from build123d import *

# Parameters (mm, degrees)
SKETCH_1_W          = 66
SKETCH_1_H          = 80
EXTRUDE_1_DEPTH     = 6
SKETCH_2_W          = 41.2
SKETCH_2_H          = 64.2
CUT_EXTRUDE_1_DEPTH = 3
FILLET_1_R          = 1
SKETCH_3_R          = 2.1
CUT_EXTRUDE_2_DEPTH = 53.201532545
CHAMFER_1_SIZE      = 1
FILLET_2_R          = 20
FILLET_3_R          = 10
CHAMFER_2_SIZE      = 1


with BuildPart() as part:
    # Эскиз1 → Бобышка-Вытянуть1 (new body)
    with BuildSketch(Plane(origin=(0, 0, 0), x_dir=(1, 0, 0), z_dir=(0, 1, 0))):
        Rectangle(SKETCH_1_W, SKETCH_1_H)
    extrude(amount=EXTRUDE_1_DEPTH)

    # Эскиз2 → Вырез-Вытянуть1 (cut)
    with BuildSketch(Plane(origin=(0, 6, 0), x_dir=(1, 0, 0), z_dir=(0, 1, 0))):
        with Locations((0, -4.1)):
            Rectangle(SKETCH_2_W, SKETCH_2_H)
    extrude(amount=-CUT_EXTRUDE_1_DEPTH, mode=Mode.SUBTRACT)

    # Скругление1
    fillet_1_edges = [part.edges().sort_by_distance(p)[0] for p in [
        (20.6, 4.5, -28),
        (20.6, 4.5, 36.2),
        (-20.6, 4.5, 36.2),
        (-20.6, 4.5, -28),
        (20.6, 6, 4.1),
        (0, 6, -28),
        (-20.6, 6, 4.1),
        (0, 6, 36.2),
    ]]
    fillet(fillet_1_edges, radius=FILLET_1_R)

    # Эскиз3 → Вырез-Вытянуть2 (cut, through all)
    with BuildSketch(Plane(origin=(0, 6, 0), x_dir=(1, 0, 0), z_dir=(0, 1, 0))):
        with Locations(Location((0, 34, 0), (0, 0, 270))):
            Circle(SKETCH_3_R)
        with Locations(Location((-29.5, 4.5, 0), (0, 0, 270))):
            Circle(SKETCH_3_R)
        with Locations(Location((29.5, 4.5, 0), (0, 0, 270))):
            Circle(SKETCH_3_R)
    extrude(amount=-CUT_EXTRUDE_2_DEPTH, mode=Mode.SUBTRACT)

    # Фаска1
    chamfer_1_edges = [part.edges().sort_by_distance(p)[0] for p in [
        (0, 6, -36.1),
        (-29.5, 6, -6.6),
        (29.5, 6, -6.6),
    ]]
    chamfer(chamfer_1_edges, length=CHAMFER_1_SIZE)

    # Скругление2
    fillet_2_edges = [part.edges().sort_by_distance(p)[0] for p in [
        (-33, 3, -40),
        (33, 3, -40),
    ]]
    fillet(fillet_2_edges, radius=FILLET_2_R)

    # Скругление3
    fillet_3_edges = [part.edges().sort_by_distance(p)[0] for p in [
        (33, 3, 40),
        (-33, 3, 40),
    ]]
    fillet(fillet_3_edges, radius=FILLET_3_R)

    # Фаска2
    # the kernel refuses this chamfer: 1 mm, written as the material it takes off along each edge
    with BuildSketch(Plane(origin=(-23, 0, 30), x_dir=(-1, 0, 0), z_dir=(0, 0, -1))) as chamfer_2_piece_1:
        Polygon((10, CHAMFER_2_SIZE), (10 - CHAMFER_2_SIZE, 0), (10, 0), align=None)
    revolve(axis=Axis((-23, 0, 30), (0, 1, 0)), revolution_arc=90, mode=Mode.SUBTRACT)
    with BuildSketch(Plane(origin=(0, 0, -34), x_dir=(0, 0, 1), z_dir=(-1, 0, 0))) as chamfer_2_piece_2:
        Polygon((2.1 + CHAMFER_2_SIZE, 0), (2.1, CHAMFER_2_SIZE), (2.1, 0), align=None)
    revolve(axis=Axis((0, 0, -34), (0, 1, 0)), mode=Mode.SUBTRACT)
    with BuildSketch(Plane(origin=(-29.5, 0, -4.5), x_dir=(0, 0, 1), z_dir=(-1, 0, 0))) as chamfer_2_piece_3:
        Polygon((2.1 + CHAMFER_2_SIZE, 0), (2.1, CHAMFER_2_SIZE), (2.1, 0), align=None)
    revolve(axis=Axis((-29.5, 0, -4.5), (0, 1, 0)), mode=Mode.SUBTRACT)
    with BuildSketch(Plane(origin=(29.5, 0, -4.5), x_dir=(0, 0, 1), z_dir=(-1, 0, 0))) as chamfer_2_piece_4:
        Polygon((2.1 + CHAMFER_2_SIZE, 0), (2.1, CHAMFER_2_SIZE), (2.1, 0), align=None)
    revolve(axis=Axis((29.5, 0, -4.5), (0, 1, 0)), mode=Mode.SUBTRACT)
    with BuildSketch(Plane(origin=(-33, 0, -20), x_dir=(-0.02749587661058908, 0.9996219169112968, 0), z_dir=(0, 0, 1)), Plane(origin=(33, 0, 30), x_dir=(0.02749587661058908, 0.9996219169112968, 0), z_dir=(0, 0, -1))) as chamfer_2_piece_5:
        Polygon((CHAMFER_2_SIZE * 0.999621916911, -CHAMFER_2_SIZE * 0.0274958766106), (-CHAMFER_2_SIZE * 0.0274958766106, -CHAMFER_2_SIZE * 0.999621916911), (0, 0), align=None)
    extrude(amount=50, mode=Mode.SUBTRACT)
    with BuildSketch(Plane(origin=(13, 0, -40), x_dir=(0, 0.9996219169112968, -0.02749587661058908), z_dir=(-1, 0, 0))) as chamfer_2_piece_6:
        Polygon((CHAMFER_2_SIZE * 0.999621916911, -CHAMFER_2_SIZE * 0.0274958766106), (-CHAMFER_2_SIZE * 0.0274958766106, -CHAMFER_2_SIZE * 0.999621916911), (0, 0), align=None)
    extrude(amount=26, mode=Mode.SUBTRACT)
    with BuildSketch(Plane(origin=(13, 0, -20), x_dir=(1, 0, 0), z_dir=(0, 0, 1))) as chamfer_2_piece_7:
        Polygon((20, CHAMFER_2_SIZE), (20 - CHAMFER_2_SIZE, 0), (20, 0), align=None)
    revolve(axis=Axis((13, 0, -20), (0, 1, 0)), revolution_arc=90, mode=Mode.SUBTRACT)
    with BuildSketch(Plane(origin=(-13, 0, -20), x_dir=(-1, 0, 0), z_dir=(0, 0, 1))) as chamfer_2_piece_8:
        Polygon((20, -CHAMFER_2_SIZE), (20 - CHAMFER_2_SIZE, 0), (20, 0), align=None)
    revolve(axis=Axis((-13, 0, -20), (0, -1, 0)), revolution_arc=90, mode=Mode.SUBTRACT)
    with BuildSketch(Plane(origin=(-23, 0, 40), x_dir=(0, 0.9996219169112968, 0.02749587661058908), z_dir=(1, 0, 0))) as chamfer_2_piece_9:
        Polygon((CHAMFER_2_SIZE * 0.999621916911, -CHAMFER_2_SIZE * 0.0274958766106), (-CHAMFER_2_SIZE * 0.0274958766106, -CHAMFER_2_SIZE * 0.999621916911), (0, 0), align=None)
    extrude(amount=46, mode=Mode.SUBTRACT)
    with BuildSketch(Plane(origin=(23, 0, 30), x_dir=(0, 0, 1), z_dir=(-1, 0, 0))) as chamfer_2_piece_10:
        Polygon((10, CHAMFER_2_SIZE), (10 - CHAMFER_2_SIZE, 0), (10, 0), align=None)
    revolve(axis=Axis((23, 0, 30), (0, 1, 0)), revolution_arc=90, mode=Mode.SUBTRACT)


solid = part.part
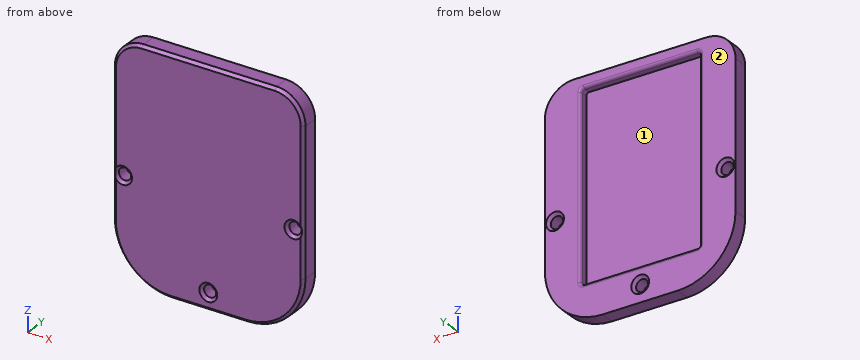
Read the model definition and answer for the solid it produces. Units are mm, in the model's axes. Face numbers are marked on the shaded views. A direction names the side the tool comes from. Round coordinates to 2 decimals unless told otherwise and drop trailing zeros. Loops run counter-clockwise (first coordinate to the right, second up) from the corner with the lowest first, then second, coordinate; pieces in that order, holes last.
Q1. Each of these flat-tipped pins is pushed along its axis until it touches: pin 1 (5 mm diameter, centred on x = -12, z = 18, fed in from +Y); pin 2 (6 mm diameter, centred on x = 17.5, z = -9, fed in from -Y); pin 3 (5 mm diameter, centred on x = 29.5, z = -4.5, fed in from -Y). Where does it stop, or does it pass through?
Q2. Consider probe 1 along X at (y, z) = (2.35, -4.5); probe 2 along X at (y, z) = (3.95, -4.5); probe 3 along X at (y, z) = (3.5, 23). Determine where each line is inside the solid, lowest interval first.
Q3. Section C-C on x = -9.5 is taken. Write down the section's boundary in (y, z), and give its area (3 significant figures).
Q4. Section B-B on z = -4.5 is taken. Write down the section's boundary in (x, y).
Q5. Which of the six approach directions +Z, -Z, +X, -X, +Y, -Y give full straight-line access (tool end or side, diameter ignored) to the marked faces 1 and 2?
Q6. Section A-A on x = 0 is taken. Write down the section's boundary in (y, z).
Q7. Section D-D on z = 28 is taken. Write down the section's boundary in (x, y).
Output:
1. pin 1: stops at y = 3
1. pin 2: stops at y = 0
1. pin 3: stops at y = 0.6
2. probe 1: x = -33 to -31.6, -27.4 to 27.4, 31.6 to 33
2. probe 2: x = -33 to -31.6, -27.4 to -20.6, 20.6 to 27.4, 31.6 to 33
2. probe 3: x = -33 to -20.6, 20.6 to 33
3. outline: (0, -39) - (1, -40) - (6, -40) - (6, -29) arc R1 ccw to (5, -28) - (3, -28) - (3, 36.2) - (5, 36.2) arc R1 ccw to (6, 37.2) - (6, 40) - (1, 40) - (0, 39) - close
3. area: 286 mm2
4. outline: (-33, 1) - (-32.3, 0.3) - (-31.6, 1) - (-31.6, 5) - (-32.6, 6) - (-33, 6) - close; (-27.4, 1) - (-26.4, 0) - (26.4, 0) - (27.4, 1) - (27.4, 5) - (26.4, 6) - (21.6, 6) arc R1 ccw to (20.6, 5) - (20.6, 3) - (-20.6, 3) - (-20.6, 5) arc R1 ccw to (-21.6, 6) - (-26.4, 6) - (-27.4, 5) - close; (31.6, 1) - (32.3, 0.3) - (33, 1) - (33, 6) - (32.6, 6) - (31.6, 5) - close
5. face 1: +Y
5. face 2: +Z, -Z, +X, -X, +Y
6. outline: (0, -39) - (1, -40) - (6, -40) - (6, -37.1) - (5, -36.1) - (1, -36.1) - (0, -37.1) - close; (0, -30.9) - (1, -31.9) - (5, -31.9) - (6, -30.9) - (6, -29) arc R1 ccw to (5, -28) - (3, -28) - (3, 36.2) - (5, 36.2) arc R1 ccw to (6, 37.2) - (6, 40) - (1, 40) - (0, 39) - close
7. outline: (-33, 1) - (-32, 0) - (32, 0) - (33, 1) - (33, 6) - (21.6, 6) arc R1 ccw to (20.6, 5) - (20.6, 3) - (-20.6, 3) - (-20.6, 5) arc R1 ccw to (-21.6, 6) - (-33, 6) - close
